Geometry check sheet. Reference: the model listing, model coordinates, mm. Face numbers are marked on the shaded views. A direction names the side the tool comes from. Give positions to 0.01 mm unless a question says otherwise; leave off trailing zeros. Loops run counter-clockwise (first coordinate to the right, second up) from the corner with the lowest first, then second, coordinate; pieces in that order, holes last.
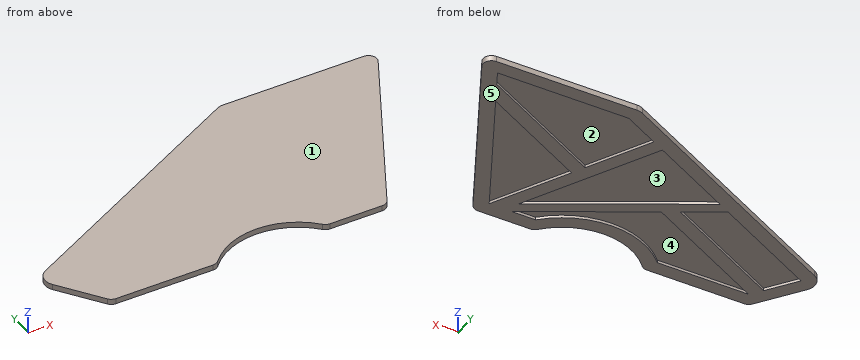
```python
from build123d import *

# Parameters (mm, degrees)
F1_DEPTH = 2
F2_DEPTH = 1


# Not quite as in the source:
# - a feature names something its author has since deleted; it is built from what else it names


with BuildPart() as f1:
    # F0 (on Top) → F1 (new body)
    with BuildSketch(Plane.XY):
        with BuildLine():
            ThreePointArc((5.132071007, 2.6840715959), (2.5813003046, -0.6052114789), (3.40420502, -4.6854862431))
            Line((3.40420502, -4.6854862431), (14.383941925, -19.7977976106))
            ThreePointArc((14.383941925, -19.7977976106), (15.4490214089, -20.7074614263), (16.8109929081, -21.0344418537))
            Line((16.8109929081, -21.0344418537), (51.8963127054, -21.0344418537))
            ThreePointArc((51.8963127054, -21.0344418537), (53.12065768, -20.7732334455), (54.1317965199, -20.035094776))
            ThreePointArc((54.1317965199, -20.035094776), (73.0425506447, -11.4896803777), (92.0885582947, -19.7292387035))
            ThreePointArc((92.0885582947, -19.7292387035), (93.0892746148, -20.4413889466), (94.2915113407, -20.6928208003))
            Line((94.2915113407, -20.6928208003), (113.1330302084, -20.6928208003))
            ThreePointArc((113.1330302084, -20.6928208003), (114.6781444331, -20.2643227024), (115.781872987, -19.1012354886))
            Line((115.781872987, -19.1012354886), (150.1493414199, 45.5345719401))
            ThreePointArc((150.1493414199, 45.5345719401), (150.0720005434, 48.4881008532), (147.5004986413, 49.9429866284))
            Line((147.5004986413, 49.9429866284), (96.7218968968, 49.9429866284))
            ThreePointArc((96.7218968968, 49.9429866284), (95.5288247883, 49.7985585766), (94.4046779119, 49.373618206))
            Line((94.4046779119, 49.373618206), (5.132071007, 2.6840715959))
        make_face()
        with BuildLine():
            Line((83.7633376258, 38.1656639161), (96.7218969194, 44.9429865363))
            Line((96.7218969194, 44.9429865363), (144.1719395233, 44.9429865363))
            Line((144.1719395233, 44.9429865363), (141.3464313092, 39.6289784601))
            Line((141.3464313092, 39.6289784601), (137.1905609573, 31.8129231027))
            Line((137.1905609573, 31.8129231027), (111.931308915, -15.6928207082))
            Line((111.931308915, -15.6928207082), (103.8109142352, -15.6928207082))
            Line((103.8109142352, -15.6928207082), (95.14885507, -15.6928207082))
            ThreePointArc((95.14885507, -15.6928207082), (73.0119644332, -6.489765959), (51.0202089869, -16.0344417616))
            Line((51.0202089869, -16.0344417616), (18.1341059978, -16.0344417616))
            Line((18.1341059978, -16.0344417616), (17.830043854, -16.0344417616))
            Line((17.830043854, -16.0344417616), (14.9430452948, -12.0608291403))
            Line((14.9430452948, -12.0608291403), (7.4492901291, -1.7465600138))
            Line((7.4492901291, -1.7465600138), (45.2243497545, 18.0097848295))
            Line((45.2243497545, 18.0097848295), (49.4777560689, 20.234315055))
            Line((49.4777560689, 20.234315055), (79.3327060482, 35.8484449312))
            Line((79.3327060482, 35.8484449312), (83.7633376258, 38.1656639161))
        make_face(mode=Mode.SUBTRACT)
        Polygon((144.1719395233, 44.9429865363), (96.7218969194, 44.9429865363), (83.7633376258, 38.1656639161), (95.5301042855, 15.6670531815), (141.3464313092, 39.6289784601), align=None)
        Polygon((103.8606077396, -11.0500555872), (79.3327060482, 35.8484449312), (49.4777560689, 20.234315055), align=None)
        Polygon((58.1843801115, 10.554375987), (45.2243497545, 18.0097848295), (7.4492901291, -1.7465600138), (14.9430452948, -12.0608291403), align=None)
        Polygon((95.5301042855, 15.6670531815), (83.7633376258, 38.1656639161), (79.3327060482, 35.8484449312), (103.8606077396, -11.0500555872), (49.4777560689, 20.234315055), (45.2243497545, 18.0097848295), (58.1843801115, 10.554375987), (14.9430452948, -12.0608291403), (17.830043854, -16.0344417616), (18.1341059978, -16.0344417616), (63.3220791259, 7.5988546181), (103.8109142352, -15.6928207082), (111.931308915, -15.6928207082), (97.8473232704, 11.236421604), (137.1905609573, 31.8129231027), (141.3464313092, 39.6289784601), align=None)
        with BuildLine():
            Line((95.14885507, -15.6928207082), (103.8109142352, -15.6928207082))
            Line((103.8109142352, -15.6928207082), (63.3220791259, 7.5988546181))
            Line((63.3220791259, 7.5988546181), (18.1341059978, -16.0344417616))
            Line((18.1341059978, -16.0344417616), (51.0202089869, -16.0344417616))
            ThreePointArc((51.0202089869, -16.0344417616), (73.0119644332, -6.489765959), (95.14885507, -15.6928207082))
        make_face()
        Polygon((111.931308915, -15.6928207082), (137.1905609573, 31.8129231027), (97.8473232704, 11.236421604), align=None)
    extrude(amount=F1_DEPTH)

    # F0 (on Top) → F2 (cut)
    with BuildSketch(Plane.XY):
        Polygon((144.1719395233, 44.9429865363), (96.7218969194, 44.9429865363), (83.7633376258, 38.1656639161), (95.5301042855, 15.6670531815), (141.3464313092, 39.6289784601), align=None)
        Polygon((103.8606077396, -11.0500555872), (79.3327060482, 35.8484449312), (49.4777560689, 20.234315055), align=None)
        Polygon((111.931308915, -15.6928207082), (137.1905609573, 31.8129231027), (97.8473232704, 11.236421604), align=None)
        Polygon((58.1843801115, 10.554375987), (45.2243497545, 18.0097848295), (7.4492901291, -1.7465600138), (14.9430452948, -12.0608291403), align=None)
        with BuildLine():
            Line((95.14885507, -15.6928207082), (103.8109142352, -15.6928207082))
            Line((103.8109142352, -15.6928207082), (63.3220791259, 7.5988546181))
            Line((63.3220791259, 7.5988546181), (18.1341059978, -16.0344417616))
            Line((18.1341059978, -16.0344417616), (51.0202089869, -16.0344417616))
            ThreePointArc((51.0202089869, -16.0344417616), (73.0119644332, -6.489765959), (95.14885507, -15.6928207082))
        make_face()
    extrude(amount=F2_DEPTH, mode=Mode.SUBTRACT)


solid = f1.part
```
1) Scan lines: line 1 along Y through (x, z) = (31, 0.9); line 2 along Y through (x, z) = (27.5, 0.4); line 3 along X through (y, z) = (26.5, 0.9). Record each from-to range of solid material in increasing order.
2) Sectioned sample at A-A on z = 1.45. Enter the section's corners in (x, y), plus the area to 3 significant figures.
3) Depth check by flat-ended pin: P1, Ø19, axis at x = 55, y = -1.5, coming from the -Z side; P2, Ø6, axis at x = 111, y = 33, coming from the -Z side; P3, Ø0.8, axis at x = 123.5, z = 0.5, coming from the -Y side; P4, Ø1.1, axis at x = 28.5, z = 0.5, coming from the +Y side. Enter the tip coordinate at first touch or a pass-through.
4) Tool access check on the marked faces 1 and 2. Record the directions out of +Z, -Z, +X, -X, +Y, -Y that give a thin tool (end or side, any length) a straight path to the whole face; none if there is none.
5) Mould release check, pull along Y, two halves, no side actions. Record for the marked faces 3, 4 and 5: +Y half, -Y half, draft (parallel to the pull), parting line (faces both ways), or undercut.
6) Sectioned sample at B-B on y = 5. Enter the section's corners in (x, z), plus the area to 3 significant figures.
7) Sectioned sample at D-D on y = 14. Enter the section's corners in (x, z), plus the area to 3 significant figures.
8) Sectioned sample at C-C on x = 75. Enter the section's corners in (y, z).
Determined:
1. line 1: y = -21.03 to -16.03, -9.31 to -3.66, 10.57 to 16.21
1. line 2: y = -21.03 to -16.03, -11.14 to -5.49, 8.74 to 14.38
1. line 3: x = 50.67 to 61.46, 84.22 to 89.86, 116.24 to 127.03, 134.37 to 140.03
2. outline: (3.4, -4.69) - (14.38, -19.8) arc R3 ccw to (16.81, -21.03) - (51.9, -21.03) arc R3 ccw to (54.13, -20.04) arc R25.66 cw to (92.09, -19.73) arc R3 ccw to (94.29, -20.69) - (113.13, -20.69) arc R3 ccw to (115.78, -19.1) - (150.15, 45.53) arc R3 ccw to (147.5, 49.94) - (96.72, 49.94) arc R5 ccw to (94.4, 49.37) - (5.13, 2.68) arc R5 ccw to start
2. area: 6,650 mm2
3. P1: stops at z = 0
3. P2: stops at z = 1
3. P3: stops at y = -5.34
3. P4: stops at y = 15.19
4. face 1: +Z, +X, -X, +Y, -Y
4. face 2: -Z
5. face 3: undercut
5. face 4: undercut
5. face 5: draft
6. outline: (9.56, 0) - (20.35, 0) - (20.35, 1) - (47.56, 1) - (47.56, 0) - (58.35, 0) - (58.35, 1) - (67.84, 1) - (67.84, 0) - (75.96, 0) - (75.96, 1) - (95.47, 1) - (95.47, 0) - (101.11, 0) - (101.11, 1) - (122.93, 1) - (122.93, 0) - (128.6, 0) - (128.6, 2) - (9.56, 2) - close
6. area: 160 mm2
7. outline: (26.77, 0) - (37.56, 0) - (37.56, 1) - (52.19, 1) - (52.19, 0) - (60.32, 0) - (60.32, 1) - (90.76, 1) - (90.76, 0) - (103.13, 0) - (103.13, 1) - (127.72, 1) - (127.72, 0) - (133.38, 0) - (133.38, 2) - (26.77, 2) - close
7. area: 144 mm2
8. outline: (-11.55, 0) - (-6.54, 0) - (-6.54, 1) - (0.88, 1) - (0.88, 0) - (5.55, 0) - (5.55, 1) - (33.58, 1) - (33.58, 0) - (39.22, 0) - (39.22, 2) - (-11.55, 2) - close
